CAD build for the part. Positions are in the model's coordinates, mm. A direction names the side the tool comes from. Coordinates: 2 decimals unless noted, no trailing zeros. Write each loop counter-clockwise with the first axis right and the second up, starting at its lowest first coordinate (ties: lowest second). Pieces come first, ordered by that corner, then holes. Notation, with made-up numbers: (-22, -26.5) - (30, -26.5) arc R29 ccw to (30, 2.5) - close; hole circle Ø6 at (24.25, 16.5). An arc over 180 degrees is marked (long way). One line per question, with ' | ' between items. Start each with the question number.
1. Flat gauge pin, fed straight in: P1, Ø4, axis at x = -35.5, y = -10, coming from the -Z side. Where does the tip first touch, or does it go through?
2. Band-saw the part on D-D, the plane z = 17.5. Write the cut outline in (x, y), then the cut area to 3 significant figures.
3. Band-saw the part on A-A, the plane y = -12.5. Write the cut outline in (x, z).
4. Band-saw the part on B-B, the plane z = 33. Write the cut outline in (x, y).
5. Two-plate mould, pull along Z, no slides. Class faces 1 (the flat face through (-52.137, -12.325, 16.605)), 2 (the flat face through (-1.408, -12.325, 13.965)), 3 (the flat face through (74.254, -12, 37)), 4 (the flat face through (-6, 0, 33)): +Z half, -Z half, draft (parallel to the pull), parting line (faces both ways), or undercut.
6. Probe line 1 (X direction, y = -11.5, z = 46); line 2 (X direction, y = -19, z = 29); line 3 (X direction, y = -10.5, z = 30). List the from-to ranges inside material, lowest first.
7. Band-saw the part on C-C, the plane x = 1.5. Write the cut outline in (y, z), then the cut area to 3 significant figures.
8. Which spindle directions (+Z, -Z, +X, -X, +Y, -Y) get a long thin tool onto all of the face, cutting with end or side? Do faces 5 (the flat face through (-11.13, -12.32, 13.45)), 6 (the flat face through (-6, -25, 33)), 7 (the flat face through (-7, -12, 47.267)). Say none if no direction does.
from build123d import *

# Parameters (mm, degrees)
F1_DEPTH = 25


with BuildPart() as f1:
    # F0 (on Front) → F1 (new body)
    with BuildSketch(Plane.XZ):
        Polygon((78.72085, 52.266717), (-6.27915, 52.266717), (-46.589765, 52.266717), (-48.77915, 52.266717), (-91.27915, 52.266717), (-91.27915, 22.266717), (-15.959248, 1.38831), (-6.166846, 25.853948), (3.485681, 1.737779), (3.685383, 1.328899), (3.988301, 1.488861), (78.945459, 22.266717), (79.253574, 22.671859), (79.253574, 52.266717), align=None)
        Polygon((74.253574, 26.154683), (6.604014, 7.402467), (-1.91518, 28.687084), (-6.166846, 39.309575), (-10.418511, 28.687084), (-18.937705, 7.402467), (-86.27915, 26.069274), (-86.27915, 47.266717), (-6.27915, 47.266717), (74.253574, 47.266717), align=None, mode=Mode.SUBTRACT)
    extrude(amount=F1_DEPTH)


solid = f1.part
Filled in:
1) P1: stops at z = 6.25
2) outline: (-74.08, -25) - (-55.37, -25) - (-55.37, 0) - (-74.08, 0) - close; (-14.9, -25) - (-9.51, -25) - (-9.51, 0) - (-14.9, 0) - close; (-2.82, -25) - (2.56, -25) - (2.56, 0) - (-2.82, 0) - close; (43.03, -25) - (61.75, -25) - (61.75, 0) - (43.03, 0) - close | area: 1,210 mm²
3) outline: (-91.28, 22.27) - (-15.96, 1.39) - (-6.17, 25.85) - (3.49, 1.74) - (3.69, 1.33) - (3.99, 1.49) - (78.95, 22.27) - (79.25, 22.67) - (79.25, 52.27) - (-91.28, 52.27) - close; hole (-86.28, 26.07) - (-18.94, 7.4) - (-6.17, 39.31) - (6.6, 7.4) - (74.25, 26.15) - (74.25, 47.27) - (-86.28, 47.27) - close
4) outline: (-91.28, -25) - (-86.28, -25) - (-86.28, 0) - (-91.28, 0) - close; (-8.69, -25) - (-3.64, -25) - (-3.64, 0) - (-8.69, 0) - close; (74.25, -25) - (79.25, -25) - (79.25, 0) - (74.25, 0) - close
5) face 1: undercut | face 2: -Z half | face 3: undercut | face 4: draft
6) line 1: x = -91.28 to -86.28, 74.25 to 79.25 | line 2: x = -91.28 to -86.28, -10.29 to -2.04, 74.25 to 79.25 | line 3: x = -91.28 to -86.28, -9.89 to -2.44, 74.25 to 79.25
7) outline: (-25, 6.7) - (0, 6.7) - (0, 20.15) - (-25, 20.15) - close; (-25, 47.27) - (0, 47.27) - (0, 52.27) - (-25, 52.27) - close | area: 461 mm²
8) face 5: -Z, +Y, -Y | face 6: +Z, -Z, +X, -X, -Y | face 7: +Y, -Y
